Input: dimensioned drawing with shaded views. Units: mm. Origin: part minimum x, y, z. Round coordinates to 2 decimals unless told otherwise and drop trailing zeros. Loops run counter-clockwise (first coordinate to the right, second up) from the corner with the lowest first, then second, coordinate; pieces in that order, holes last. Notation, with made-up numbers: (-7.75, -14.75) - (26.25, -14.75) arc R30 cw to (26.25, 14.25) - close; hole circle Ø6 at (-25.75, 14). An arc over 180 degrees is marked (long way). One line per question, with ' | ' between items. Start each with the question number.
1. Cut plane A-A (x = 4). Return loops of the section in (y, z), then the cut area to 3 significant figures.
2. Mould query, pull axis Y, two halves, no side actions, for the marked faces 1, 2 and 3. Classes: pulls with the +Y half, pulls with the -Y half, needs draft (parallel to the pull), parting line crosses it, or undercut.
3. Cut plane D-D (z = 1.95). Return loops of the section in (x, y), then the cut area to 3 significant figures.
4. Ray query, line 1 (Y direction, x = 4, z = 2.75); line 2 (Y direction, x = 31, z = 3.2); line 3 (Y direction, x = 21.5, z = 3.35). Return the intervals inside material, ascending.
5. Cut plane B-B (y = 31). Return loops of the section in (x, z).
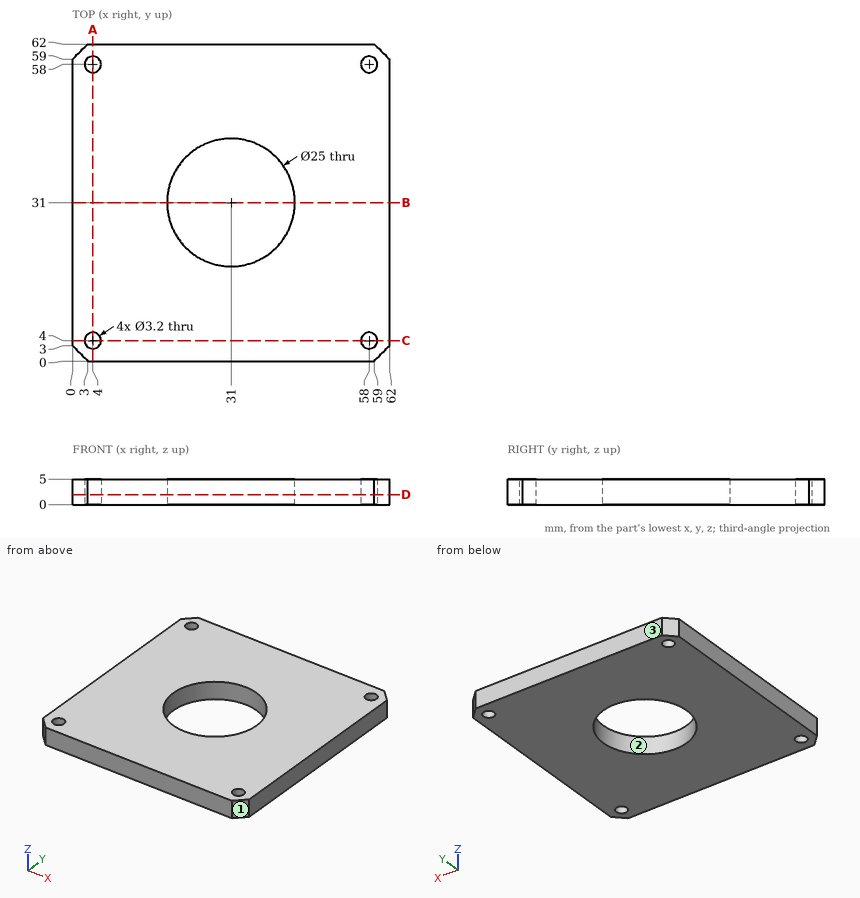
Answers follow:
1) outline: (0, 0) - (2.4, 0) - (2.4, 5) - (0, 5) - close; (5.6, 0) - (56.4, 0) - (56.4, 5) - (5.6, 5) - close; (59.6, 0) - (62, 0) - (62, 5) - (59.6, 5) - close | area: 278 mm2
2) face 1: pulls with the -Y half | face 2: undercut | face 3: pulls with the +Y half
3) outline: (0, 3) - (3, 0) - (59, 0) - (62, 3) - (62, 59) - (59, 62) - (3, 62) - (0, 59) - close; hole circle Ø3.2 at (4, 4); hole circle Ø3.2 at (4, 58); hole circle Ø25 at (31, 31); hole circle Ø3.2 at (58, 4); hole circle Ø3.2 at (58, 58) | area: 3,300 mm2
4) line 1: y = 0 to 2.4, 5.6 to 56.4, 59.6 to 62 | line 2: y = 0 to 18.5, 43.5 to 62 | line 3: y = 0 to 22.88, 39.12 to 62
5) outline: (0, 0) - (18.5, 0) - (18.5, 5) - (0, 5) - close; (43.5, 0) - (62, 0) - (62, 5) - (43.5, 5) - close
